```python
from build123d import *

# Parameters (mm, degrees)
SKETCH1_R           = 5
SKETCH1_W           = 35
SKETCH1_H           = 20
BOSS_EXTRUDE1_DEPTH = 12
SKETCH1_3_R         = 5
BOSS_EXTRUDE2_DEPTH = 25


with BuildPart() as part:
    # Sketch1 → Boss-Extrude1 (new body)
    with BuildSketch(Plane(origin=(0, 0, 0), x_dir=(1, 0, 0), z_dir=(0, 1, 0))):
        Circle(SKETCH1_R)
        Rectangle(SKETCH1_W, SKETCH1_H)
        Circle(SKETCH1_R, mode=Mode.SUBTRACT)
    extrude(amount=BOSS_EXTRUDE1_DEPTH)

    # Sketch1_3 → Boss-Extrude2 (add)
    with BuildSketch(Plane(origin=(0, 0, 0), x_dir=(1, 0, 0), z_dir=(0, 1, 0))):
        Circle(SKETCH1_3_R)
    extrude(amount=BOSS_EXTRUDE2_DEPTH)


solid = part.part
```
Check sheet for the modelled part. Datum: model origin and axes. Units: mm. A direction names the side the tool comes from. Round coordinates to 2 decimals unless told otherwise and drop trailing zeros. Order: outer loops, then holes, each group sorted by start corner. A loop starts at its lowest first (then second) coordinate and runs counter-clockwise, first axis right, second up. Notation, with made-up numbers: M 69,16.5 L 76,16.5 A10 cw 76,32.5 Z; hole C 28.5,-29 d9. An arc over 180 degrees is marked long. Answer in a Markdown table with one row per item.
(1) Section check B-B on z = -4.25. Record the boundary of the cut face in (x, y), plus the area to 3 significant figures.
Findings:
| item | result |
|---|---|
| outline | M -17.5,0 L 17.5,0 L 17.5,12 L 2.63,12 L 2.63,25 L -2.63,25 L -2.63,12 L -17.5,12 Z |
| area | 488 mm^2 |
(2) Section check D-D on z = 6.5. Record the boundary of the cut face in (x, y).
Findings:
| item | result |
|---|---|
| outline | M -17.5,0 L 17.5,0 L 17.5,12 L -17.5,12 Z |
(3) Gauge pin test, flat ends, axial feed: pin 1 (2 mm diameter, centred on x = -4.5, y = 14, fed in from -Z); pin 2 (1 mm diameter, centred on x = -6.5, z = 3, fed in from +Y). Record the tip position at first contact, or that the pin passes through.
Findings:
| item | result |
|---|---|
| pin 1 | stops at z = -3.57 |
| pin 2 | stops at y = 12 |
(4) Section check C-C on y = 12.5. Record the boundary of the cut face in (x, z).
Findings:
| item | result |
|---|---|
| outline | C 0,0 d10 |
(5) Section check A-A on x = 0. Record the boundary of the cut face in (y, z).
Findings:
| item | result |
|---|---|
| outline | M 0,-10 L 12,-10 L 12,-5 L 25,-5 L 25,5 L 12,5 L 12,10 L 0,10 Z |
(6) Set-up check for faces 1 (the flat face through (0, 6, -10)), 2 (the cylindrical face through (-1.08, 18.41, 4.88)): record each of +Z, -Z, +X, -X, +Y, -Y from which the full face is reachable in a straight line by a thin tool's end or side.
Findings:
| item | result |
|---|---|
| face 1 | -Z, +X, -X, +Y, -Y |
| face 2 | +Y |
(7) Material ranges on line 1 along Y through (x, z) = (0, 6); line 2 along X through (y, z) = (23.5, 0.25); line 3 along Z through (x, y) = (0, 13), recorded low to high. Write a range as from..to.
Findings:
| item | result |
|---|---|
| line 1 | y = 0..12 |
| line 2 | x = -4.99..4.99 |
| line 3 | z = -5..5 |
